For this review, take the finished solid that the model builds, in its own axes (mm). A direction names the side the tool comes from. Round coordinates to 2 decimals unless told otherwise and drop trailing zeros. Order: outer loops, then holes, each group sorted by start corner. A loop starts at its lowest first (then second) coordinate and runs counter-clockwise, first axis right, second up. Notation, with made-up numbers: (-2.5, 68) - (25.5, 68) arc R22 ccw to (25.5, 107) - close; hole circle Ø10 at (2.25, 38). An arc over 180 degrees is marked (long way). One line per question, with ' | ' between items.
```python
from build123d import *

# Parameters (mm, degrees)
F0_R        = 4.875
F0_R_2      = 2.125
F1_DEPTH    = 5
F2_R        = 4.875
F3_DEPTH    = 30
F4_T1_DEPTH = 5
F6_DEPTH    = 20
F8_DEPTH    = 15
F9_R        = 2.125
F10_DEPTH   = 40.001
F11_R       = 2.125
F12_DEPTH   = 40.001
F13_SIZE    = 5


# Not quite as in the source:
# - a fillet or chamfer that OpenCascade refuses, or shapes differently, is made with other operations: its cross-section is extruded or revolved along the edge and cut away or added


with BuildPart() as f1:
    # F0 (on Top) → F1 (new body)
    with BuildSketch(Plane.XY):
        Polygon((-12.5, 27.5), (-12.5, 0), (-12.5, -12.5), (27.5, -12.5), (27.5, 7.5), (7.5, 7.5), (7.5, 27.5), align=None)
        Circle(F0_R, mode=Mode.SUBTRACT)
        with Locations((17.5, 0)):
            Circle(F0_R_2, mode=Mode.SUBTRACT)
        with Locations((0, 17.5)):
            Circle(F0_R_2, mode=Mode.SUBTRACT)
    extrude(amount=F1_DEPTH)

    # F2 (on face) → F3 (join)
    with BuildSketch(Plane(origin=(0, 0, 0), x_dir=(1, 0, 0), z_dir=(0, 0, -1))):
        Polygon((12.5, -5.1776695297), (12.5, 5.1776695297), (5.1776695297, 12.5), (-5.1776695297, 12.5), (-12.5, 5.1776695297), (-12.5, -5.1776695297), (-5.1776695297, -12.5), (5.1776695297, -12.5), (7.5, -10.1776695297), (7.5, -7.5), (10.1776695297, -7.5), align=None)
        Circle(F2_R, mode=Mode.SUBTRACT)
        Polygon((7.5, -10.1776695297), (10.1776695297, -7.5), (7.5, -7.5), align=None)
    extrude(amount=F3_DEPTH)

    # F4: chamfer of 5 on 1 edges, made by hand

    # F4_s2 → F4_t1 (join)
    with BuildSketch(Plane.XY):
        Polygon((12.5, 7.5), (7.5, 12.5), (7.5, 7.5), align=None)
    extrude(amount=F4_T1_DEPTH)

    # F5 (on face) → F6 (join)
    with BuildSketch(Plane.XY.offset(5)):
        Polygon((-7.5, 27.5), (-12.5, 27.5), (-12.5, -12.5), (27.5, -12.5), (27.5, -7.5), (-7.5, -7.5), align=None)
    extrude(amount=F6_DEPTH)

    # F7 (on face) → F8 (join)
    with BuildSketch(Plane.XY.offset(25)):
        Polygon((-7.5, 12.5), (-12.5, 12.5), (-12.5, -12.5), (12.5, -12.5), (12.5, -7.5), (-7.5, -7.5), align=None)
    extrude(amount=F8_DEPTH)

    # F9 (on face) → F10 (cut, through all)
    with BuildSketch(Plane.XZ.offset(12.5)):
        with Locations((20, 12.5)):
            Circle(F9_R)
        with Locations((0, 32.5)):
            Circle(F9_R)
    extrude(amount=-F10_DEPTH, mode=Mode.SUBTRACT)

    # F11 (on face) → F12 (cut, through all)
    with BuildSketch(Plane(origin=(-12.5, 0, 0), x_dir=(0, -1, 0), z_dir=(-1, 0, 0))):
        with Locations((-20, 12.5)):
            Circle(F11_R)
        with Locations((0, 32.5)):
            Circle(F11_R)
    extrude(amount=-F12_DEPTH, mode=Mode.SUBTRACT)

    # F13
    f13_edges = [f1.edges().sort_by_distance(p)[0] for p in [
        (12.5, -10, 25),
        (-10, 12.5, 25),
    ]]
    chamfer(f13_edges, length=F13_SIZE)


solid = f1.part
```
(1) For faces 5 (the flat face through (-8.79, -8.89, -14.79)), 6 (the flat face through (-7.5, 6, 18)), 7 (the flat face through (-10, 12.5, 35)), 8 (the flat face through (20, 7.5, 2)), 9 (the flat face through (12.5, 0, -15)), list the 3-axis set-ups (+Z, -Z, +X, -X, +Y, -Y) from which the entire face can be reached by the end or side of a thin tool; tool diameter is ignored.
Output values:
face 5: -Z, -X, -Y | face 6: +Z, +X, +Y | face 7: +Z, +X, -X, +Y | face 8: +Z, -Z, +X, +Y | face 9: -Z, +X, +Y, -Y
(2) For probe 1 along Y at (x, z) = (0, 2) (3 decimals); probe 2 along Z at (x, y) = (-9, 0) (3 decimals); probe 3 along Z at (x, y) = (20, -10) (3 decimals), list the stretches that pass through material, from the lowest coordinate up. Write a range as [from, to].
Output values:
probe 1: [-12.5, -4.875], [4.875, 15.375], [19.625, 27.5] | probe 2: [-30, 30.375], [34.625, 40] | probe 3: [0, 10.375], [14.625, 25]
(3) We need section C-C on y = 20.5. State the section outline as (x, z) points.
Output values:
outline: (-12.5, 0) - (7.5, 0) - (7.5, 5) - (-7.5, 5) - (-7.5, 10.43) - (-12.5, 10.43) - close; (-12.5, 14.57) - (-7.5, 14.57) - (-7.5, 25) - (-12.5, 25) - close
(4) We need section B-B on x = 0. State the section outline as (y, z) points (3 decimals), plus the area to 3 significant figures.
Output values:
outline: (-12.5, -30) - (-4.875, -30) - (-4.875, 5) - (-7.5, 5) - (-7.5, 30.375) - (-12.5, 30.375) - close; (-12.5, 34.625) - (-7.5, 34.625) - (-7.5, 40) - (-12.5, 40) - close; (4.875, -30) - (12.5, -30) - (12.5, 0) - (15.375, 0) - (15.375, 5) - (4.875, 5) - close; (19.625, 0) - (27.5, 0) - (27.5, 5) - (19.625, 5) - close | area: 741 mm^2
(5) We need section D-D on y = 14.5. State the section outline as (x, z) points.
Output values:
outline: (-12.5, 0) - (7.5, 0) - (7.5, 5) - (-7.5, 5) - (-7.5, 28) - (-12.5, 28) - close
(6) Mouldability with a two-part tool opening along Z and no side actions: class faces 1 (the cylindrical face through (-0.277, 19.607, 2.465)), 2 (the cylindrical face through (-10.035, 22.123, 12.593)), 3 (the cylindrical face through (-0.461, -10.035, 30.426)), 4 (the flat face through (0, -6, -30)) as released by +Z, released by -Z, zero draft, split by the parting line, or undercut.
Output values:
face 1: zero draft | face 2: undercut | face 3: undercut | face 4: released by -Z
(7) Insertion check: pin 1 (12 mm diameter, centred on x = -6.5, z = -22.5, fed in from +Y); pin 2 (7 mm diameter, centred on x = 0, y = 17.5, fed in from -Z); pin 3 (10 mm diameter, centred on x = 16.5, z = 17.5, fed in from +Y). Each pin has a flat end and moves straight along its axis. Give the tip position at first contact, or say it passes through.
Output values:
pin 1: y = 12.5 | pin 2: z = 0 | pin 3: y = -7.5
(8) We need section A-A on z = 12.5. State the section outline as (x, y) points (3 decimals).
Output values:
outline: (-12.5, -12.5) - (17.875, -12.5) - (17.875, -7.5) - (-7.5, -7.5) - (-7.5, 17.875) - (-12.5, 17.875) - close; (-12.5, 22.125) - (-7.5, 22.125) - (-7.5, 27.5) - (-12.5, 27.5) - close; (22.125, -12.5) - (27.5, -12.5) - (27.5, -7.5) - (22.125, -7.5) - close
